Could you check a few things on this model? Use its own coordinates, in mm. Face numbers are marked on the shaded views. Give positions to 0.01 mm unless a question says otherwise; leave off trailing zeros. Write each loop counter-clockwise with the first axis right and the second up, starting at its lowest first coordinate (ties: lowest second). Pieces come first, ordered by that corner, then holes. Notation, with made-up numbers: (-12, 45.5) - (-6, 45.5) arc R26 ccw to (-6, 81.5) - close; hole circle Ø1 at (-19.5, -29). An arc over 180 degrees is marked (long way). Answer as CSV lines item,"result". Start each with the question number.
Q1. Imagine slicing it at A-A on y = 0. List the corners of the cut face in (x, z) for me.
Q2. We'd pull the mould along Y, two halves only. Please class the marked faces 1, 2 and 3: pulls with the +Y half, pulls with the -Y half, needs draft (parallel to the pull), parting line crosses it, or undercut.
Q3. Imagine slicing it at C-C on z = 7. List the corners of the cut face in (x, y) for me.
Q4. Will these pins go through, and if not, where does the flat tip stop? pin 1 Ø1 at (y, z) = (26.5, 5) entering from -X; pin 2 Ø5 at (y, z) = (-27, 3) entering from -X; pin 3 Ø4 at (x, z) = (-5, -6) entering from +Y; pin 4 Ø9 at (x, y) = (0, 0) entering from +Z.
Q5. If I drill on line 1 along Y through (x, z) = (0, 2); line 2 along Y through (x, z) = (-1.5, -8); line 3 along Y through (x, z) = (6, -7.5), over which ranges is the centre line in solid material (lowest first)?
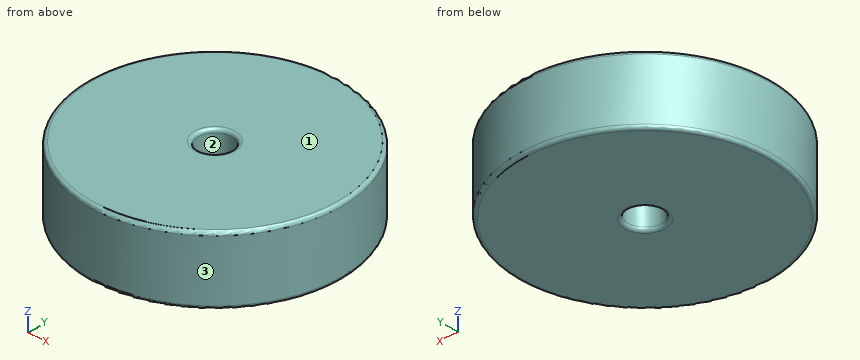
Solid Edge part; units mm, degrees
sketch "Sketch1" plane through (0, 0, 0) normal (0, 0, 1) x (1, 0, 0)
  circle A0 centre (0, 0) radius 37.5
extrude "ExtrudedProtrusion_1" add sketch "Sketch1" along normal mid plane 20
fillet "Round_1" radius 1 2 edges at (-37.5, 0, 10) (-37.5, 0, -10)
hole "Hole_1" at (0, 0, 10) direction (0, 0, -1) diameter 10 end up to next
fillet "Round_2" radius 1 2 edges at (-5, 0, 10) (5, 0, -10)
properties material "Acrylic, high impact grade"
Conclusion:
1,outline,"(-37.5, -9) arc R1 ccw to (-36.5, -10) - (-6, -10) arc R1 ccw to (-5, -9) - (-5, 9) arc R1 ccw to (-6, 10) - (-36.5, 10) arc R1 ccw to (-37.5, 9) - close; (5, -9) arc R1 ccw to (6, -10) - (36.5, -10) arc R1 ccw to (37.5, -9) - (37.5, 9) arc R1 ccw to (36.5, 10) - (6, 10) arc R1 ccw to (5, 9) - close"
2,face 1,"needs draft"
2,face 2,"undercut"
2,face 3,"parting line crosses it"
3,outline,"circle Ø75 at (0, 0); hole circle Ø10 at (0, 0)"
4,pin 1,"x = -27.02"
4,pin 2,"x = -28.39"
4,pin 3,"y = 37.38"
4,pin 4,"through"
5,line 1,"-37.5 to -5, 5 to 37.5"
5,line 2,"-37.47 to -4.77, 4.77 to 37.47"
5,line 3,"-37.02 to 37.02"
